Could you check a few things on this model? Use its own coordinates, in mm. A direction names the side the tool comes from. Coordinates: 2 decimals unless noted, no trailing zeros. Order: outer loops, then holes, each group sorted by start corner. A loop starts at its lowest first (then second) coordinate and runs counter-clockwise, first axis right, second up. Notation, with made-up numbers: (-33, 36) -> (-20, 36) arc R17 ccw to (-20, 42) -> close; hole circle Ø3 at (70.5, -14.75). An arc over 180 degrees is marked (long way). Use a Markdown table: item, result. Add a question column.
1) If we section it at B-B (x = 1.5): Write out the boundary of the cut face in (y, z), plus the area to 3 significant figures.
2) If I drill on L1, parallel to Y at x = 1.95, z = 0; L2, parallel to Y at x = 4.25, z = 7.5; L3, parallel to Z at x = 3.35, y = 6.5, over which ranges is the centre line in solid material (lowest first)? Write a range as [from, to].
3) Thinking about a two-plate mould opening in Y: for faces 1 (the cylindrical face through (2.18, -11.56, 15.08)), 2 (the flat face through (4.4, 0, 8)), 3 (the cylindrical face through (2.17, -0.42, -10.19)), which applies, +Y half, -Y half, draft (parallel to the pull), parting line (faces both ways), or undercut?
4) If we section it at C-C (z = 0): Write out the boundary of the cut face in (x, y).
5) Which directions (+Z, -Z, +X, -X, +Y, -Y) give clear straight access to the entire face, cutting with the end or side of a thin tool? Please do faces 4 (the flat face through (0, 0, 8)), 5 (the flat face through (2, 0, 7.8)).
6) Will these pins go through, and if not, where does the flat tip stop? pin 1 Ø1 at (x, z) = (3.5, 9) entering from +Y; pin 2 Ø1 at (x, z) = (3.5, 2.5) entering from +Y.
7) If we section it at A-A (y = 0): Write out the boundary of the cut face in (x, z), plus the area to 3 significant figures.
```python
from build123d import *

# Parameters (mm, degrees)
CROQUIS1_R              = 19
SALIENTE_EXTRUIR1_DEPTH = 4.4
CHAFL_N1_SIZE           = 0.6
CHAFL_N2_SIZE           = 0.6
REDONDEO1_R             = 0.4


with BuildPart() as part:
    # Croquis1 → Saliente-Extruir1 (new body)
    with BuildSketch(Plane.YZ):
        with Locations(Location((0, 0, 0), (0, 0, 270))):
            Circle(CROQUIS1_R)
        with BuildLine():
            Line((1.4, 10.103464752), (1.4, 7.8))
            Line((1.4, 7.8), (-1.4, 7.8))
            Line((-1.4, 7.8), (-1.4, 10.103464752))
            ThreePointArc((-1.4, 10.103464752), (0, -10.2), (1.4, 10.103464752))
        make_face(mode=Mode.SUBTRACT)
    extrude(amount=SALIENTE_EXTRUIR1_DEPTH)

    # Chaflán1
    chafl_n1_edges = [part.edges().sort_by_distance(p)[0] for p in [
        (0, 0, 19),
        (4.4, 0, 19),
    ]]
    chamfer(chafl_n1_edges, length=CHAFL_N1_SIZE)

    # Chaflán2
    chafl_n2_edges = [part.edges().sort_by_distance(p)[0] for p in [
        (2.2, 1.4, 7.8),
        (2.2, -1.4, 7.8),
    ]]
    chamfer(chafl_n2_edges, length=CHAFL_N2_SIZE)

    # Redondeo1
    redondeo1_edges = [part.edges().sort_by_distance(p)[0] for p in [
        (2.2, -1.4, 10.103464752),
        (2.2, 1.4, 10.103464752),
    ]]
    fillet(redondeo1_edges, radius=REDONDEO1_R)


solid = part.part
```
Answer sheet:
| question | item | result |
|---|---|---|
| 1 | outline | circle Ø38 at (0, 0); hole (-1.87, 10.03) arc R10.2 ccw (long way) to (1.87, 10.03) arc R0.4 ccw to (1.4, 9.63) -> (1.4, 8.4) -> (0.8, 7.8) -> (-0.8, 7.8) -> (-1.4, 8.4) -> (-1.4, 9.63) arc R0.4 ccw to start |
| 1 | area | 814 mm2 |
| 2 | L1 | [-19, -10.2], [10.2, 19] |
| 2 | L2 | [-16.97, -6.91], [6.91, 16.97] |
| 2 | L3 | [-17.85, -7.86], [7.86, 17.85] |
| 3 | face 1 | parting line |
| 3 | face 2 | draft |
| 3 | face 3 | undercut |
| 4 | outline | (0, -18.4) -> (0.6, -19) -> (3.8, -19) -> (4.4, -18.4) -> (4.4, -10.2) -> (0, -10.2) -> close; (0, 10.2) -> (4.4, 10.2) -> (4.4, 18.4) -> (3.8, 19) -> (0.6, 19) -> (0, 18.4) -> close |
| 5 | face 4 | +Z, -Z, -X, +Y, -Y |
| 5 | face 5 | +X, -X |
| 6 | pin 1 | y = 16.99 |
| 6 | pin 2 | y = 18.89 |
| 7 | outline | (0, -18.4) -> (0.6, -19) -> (3.8, -19) -> (4.4, -18.4) -> (4.4, -10.2) -> (0, -10.2) -> close; (0, 7.8) -> (4.4, 7.8) -> (4.4, 18.4) -> (3.8, 19) -> (0.6, 19) -> (0, 18.4) -> close |
| 7 | area | 87.3 mm2 |
